Verification items for the finished model (mm, model axes). Face numbers are marked on the shaded views. Round coordinates to 2 decimals unless told otherwise and drop trailing zeros. Loops run counter-clockwise (first coordinate to the right, second up) from the corner with the lowest first, then second, coordinate; pieces in that order, holes last. Notation, with made-up numbers: (54, -23.5) -> (100, -23.5) arc R20 ccw to (100, 9.5) -> close; hole circle Ø6 at (71.5, 77.25). An arc over 180 degrees is marked (long way). Use a Markdown table: item, result. Add a question column.
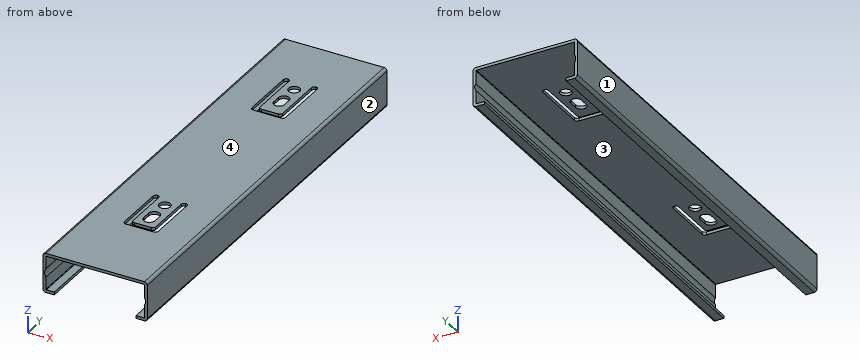
```python
from build123d import *

# Parameters (mm, degrees)
BOSS_EXTRUDE1_DEPTH = 150
FILLET1_R           = 1
FILLET2_R           = 0.2
SKETCH2_R           = 2
CUT_EXTRUDE1_DEPTH  = 155.280557534
CUT_EXTRUDE2_DEPTH  = 155.280557534
CUT_EXTRUDE3_DEPTH  = 150
FILLET7_R           = 1
SKETCH7_R           = 2
CUT_EXTRUDE4_DEPTH  = 155.280557534
CUT_EXTRUDE6_DEPTH  = 155.280557534
FILLET9_R           = 1
SKETCH12_R          = 2
SKETCH12_R_2        = 3
CUT_EXTRUDE7_DEPTH  = 155.520226026


with BuildPart() as part:
    # Sketch1 → Boss-Extrude1 (new body)
    with BuildSketch(Plane(origin=(0, 0, 0), x_dir=(1, 0, 0), z_dir=(0, 1, 0))):
        Polygon((-2.736049046, -15.431975477), (32.263950954, -15.431975477), (32.263950954, -3.431975477), (29.263950954, -3.431975477), (29.263950954, -2.431975477), (33.263950954, -2.431975477), (33.263950954, -16.431975477), (-3.736049046, -16.431975477), (-3.736049046, -2.431975477), (0.263950954, -2.431975477), (0.263950954, -3.431975477), (-2.736049046, -3.431975477), align=None)
    extrude(amount=BOSS_EXTRUDE1_DEPTH)

    # Fillet1
    fillet1_edges = [part.edges().sort_by_distance(p)[0] for p in [
        (33.263950954, 75, 2.431975477),
        (33.263950954, 75, 16.431975477),
        (-3.736049046, 75, 16.431975477),
        (-3.736049046, 75, 2.431975477),
    ]]
    fillet(fillet1_edges, radius=FILLET1_R)

    # Fillet2
    fillet2_edges = [part.edges().sort_by_distance(p)[0] for p in [
        (-2.736049046, 75, 15.431975477),
        (32.263950954, 75, 15.431975477),
        (32.263950954, 75, 3.431975477),
        (-2.736049046, 75, 3.431975477),
    ]]
    fillet(fillet2_edges, radius=FILLET2_R)

    # Sketch2 → Cut-Extrude1 (cut, through all)
    with BuildSketch(Plane.XY.offset(16.431975477)):
        with Locations((14.763950954, 124.553168405)):
            Circle(SKETCH2_R)
    extrude(amount=-CUT_EXTRUDE1_DEPTH, mode=Mode.SUBTRACT)

    # Sketch4 → Cut-Extrude2 (cut, through all)
    with BuildSketch(Plane.XY.offset(16.431975477)):
        with BuildLine():
            Line((16.632444953, 118.100326697), (16.632444953, 115.100326697))
            ThreePointArc((16.632444953, 115.100326697), (14.763950954, 113.231832698), (12.895456955, 115.100326697))
            Line((12.895456955, 115.100326697), (12.895456955, 118.100326697))
            ThreePointArc((12.895456955, 118.100326697), (14.763950954, 119.968820696), (16.632444953, 118.100326697))
        make_face()
    extrude(amount=-CUT_EXTRUDE2_DEPTH, mode=Mode.SUBTRACT)

    # Sketch6 → Cut-Extrude3 (cut)
    with BuildSketch(Plane.XY.offset(16.431975477)):
        Polygon((18.810239274, 129.292771491), (18.810239274, 109.228960099), (10.810239274, 109.228960099), (10.810239274, 129.292771491), (8.810239274, 129.292771491), (8.810239274, 107.509210665), (20.810239274, 107.509210665), (20.810239274, 129.292771491), align=None)
    extrude(amount=-CUT_EXTRUDE3_DEPTH, mode=Mode.SUBTRACT)

    # Fillet7
    fillet7_edges = [part.edges().sort_by_distance(p)[0] for p in [
        (8.810239274, 107.509210665, 15.931975477),
        (20.810239274, 107.509210665, 15.931975477),
        (18.810239274, 109.228960099, 15.931975477),
        (10.810239274, 109.228960099, 15.931975477),
        (10.810239274, 129.292771491, 15.931975477),
        (8.810239274, 129.292771491, 15.931975477),
        (18.810239274, 129.292771491, 15.931975477),
        (20.810239274, 129.292771491, 15.931975477),
    ]]
    fillet(fillet7_edges, radius=FILLET7_R - 0.0001)  # a hair under: the kernel refuses the full size

    # Sketch7 → Cut-Extrude4 (cut, through all)
    with BuildSketch(Plane.XY.offset(16.431975477)):
        with Locations((14.782730099, 43.616424241)):
            Circle(SKETCH7_R)
        with BuildLine():
            Line((16.779852756, 36.933079114), (16.778561099, 33.933079392))
            ThreePointArc((16.778561099, 33.933079392), (14.77770018, 31.933940682), (12.77856147, 33.9348016))
            Line((12.77856147, 33.9348016), (12.779853126, 36.934801322))
            ThreePointArc((12.779853126, 36.934801322), (14.780714045, 38.933940033), (16.779852756, 36.933079114))
        make_face()
    extrude(amount=-CUT_EXTRUDE4_DEPTH, mode=Mode.SUBTRACT)

    # Sketch9 → Cut-Extrude6 (cut, through all)
    with BuildSketch(Plane.XY.offset(16.431975477)):
        Polygon((18.824358564, 47.739325349), (18.824358564, 29.739325349), (10.824358564, 29.739325349), (10.824358564, 47.739325349), (8.824358564, 47.739325349), (8.824358564, 27.739325349), (20.824358564, 27.739325349), (20.824358564, 47.739325349), align=None)
    extrude(amount=-CUT_EXTRUDE6_DEPTH, mode=Mode.SUBTRACT)

    # Fillet9
    fillet9_edges = [part.edges().sort_by_distance(p)[0] for p in [
        (20.824358564, 27.739325349, 15.931975477),
        (18.824358564, 29.739325349, 15.931975477),
        (8.824358564, 27.739325349, 15.931975477),
        (10.824358564, 29.739325349, 15.931975477),
        (8.824358564, 47.739325349, 15.931975477),
        (10.824358564, 47.739325349, 15.931975477),
        (18.824358564, 47.739325349, 15.931975477),
        (20.824358564, 47.739325349, 15.931975477),
    ]]
    fillet(fillet9_edges, radius=FILLET9_R - 0.0001)  # a hair under: the kernel refuses the full size

    # Sketch12 → Cut-Extrude7 (cut, through all)
    with BuildSketch(Plane(origin=(0, 150, 0), x_dir=(1, 0, 0), z_dir=(0, 1, 0))):
        with Locations((30.665950954, -9.431975477)):
            Circle(SKETCH12_R)
        with Locations((-0.138049046, -9.431975477)):
            Circle(SKETCH12_R_2)
    extrude(amount=-CUT_EXTRUDE7_DEPTH, mode=Mode.SUBTRACT)


solid = part.part
```
1) Thickness scan on line 1 (Z direction, x = -1, y = 108); line 2 (X direction, y = 132, z = 6.5); line 3 (Z direction, x = 3.5, y = 79). Record the ranges inside material, lowest first.
2) Sectioned sample at A-A on z = 13.5. Enter the section's corners in (x, y), then the cut area to 3 significant figures.
3) Sectioned sample at C-C on x = 6. Enter the section's corners in (y, z).
4) Sectioned sample at B-B on y = 91.5. Enter the section's corners in (x, z), then the cut area to 3 significant figures.
5) Release check for a two-part mould opening along X. For the marked faces 1, 2, 3 and 4 record: released by +X, released by -X, zero draft, split by the parting line, or undercut.
6) Go/stop test with flat-tipped pins: pin 1 (0.5 mm diameter, centred on y = 41.5, z = 16, fed in from -X); pin 2 (3.5 mm diameter, centred on x = 14.76, y = 124.55, fed in from -Z); pin 3 (0.8 mm diameter, centred on y = 114, z = 16, fed in from +X). Record where each tip stops, or that it passes through.
Geometry results:
| question | item | result |
|---|---|---|
| 1 | line 1 | 2.43 to 3.43, 15.43 to 16.43 |
| 1 | line 2 | -3.74 to -2.74, 32.26 to 33.26 |
| 1 | line 3 | 15.43 to 16.43 |
| 2 | outline | (-3.74, 0) -> (-2.74, 0) -> (-2.74, 150) -> (-3.74, 150) -> close; (32.26, 0) -> (33.26, 0) -> (33.26, 150) -> (32.26, 150) -> close |
| 2 | area | 300 mm^2 |
| 3 | outline | (0, 15.43) -> (150, 15.43) -> (150, 16.43) -> (0, 16.43) -> close |
| 4 | outline | (-3.74, 3.43) arc R1 ccw to (-2.74, 2.43) -> (0.26, 2.43) -> (0.26, 3.43) -> (-2.54, 3.43) arc R0.2 cw to (-2.74, 3.63) -> (-2.74, 7.93) arc R3 cw to (-2.74, 10.93) -> (-2.74, 15.23) arc R0.2 cw to (-2.54, 15.43) -> (32.06, 15.43) arc R0.2 cw to (32.26, 15.23) -> (32.26, 10.63) arc R2 cw to (32.26, 8.23) -> (32.26, 3.63) arc R0.2 cw to (32.06, 3.43) -> (29.26, 3.43) -> (29.26, 2.43) -> (32.26, 2.43) arc R1 ccw to (33.26, 3.43) -> (33.26, 15.43) arc R1 ccw to (32.26, 16.43) -> (-2.74, 16.43) arc R1 ccw to (-3.74, 15.43) -> close |
| 4 | area | 66.7 mm^2 |
| 5 | face 1 | released by -X |
| 5 | face 2 | released by +X |
| 5 | face 3 | undercut |
| 5 | face 4 | zero draft |
| 6 | pin 1 | x = -3.68 |
| 6 | pin 2 | through |
| 6 | pin 3 | x = 33.25 |
